For this review, take the finished solid that the model builds, in its own axes (mm). Face numbers are marked on the shaded views. A direction names the side the tool comes from. Coordinates: 2 decimals unless noted, no trailing zeros. Order: outer loops, then holes, each group sorted by start corner. A loop starts at its lowest first (then second) coordinate and runs counter-clockwise, first axis right, second up. Notation, with made-up numbers: (13, 73) -> (50, 73) arc R10 cw to (50, 91) -> close; hole circle Ø3 at (-32, -6). An arc over 180 degrees is marked (long way). Return JSON: item names as keys, results as strings. Group by question number.
Item 1: Machinability: for the marked faces 1, 2, 3, 4 and 5, which of the approach directions +Z, -Z, +X, -X, +Y, -Y give a long, thin tool a straight path to every point of the face, cutting with its end or side? Answer none if there is none.
Item 2: Take a section at B-B (z = 8.5). Write out the cut boundary in (x, y) (3 decimals), then the cut area to 3 significant figures.
Item 3: For line 1 along Y through (x, z) = (-6, 7.1) (3 decimals); line 2 along X through (y, z) = (-5, 7) (3 decimals); line 3 along Z through (x, y) = (-2.5, -3), list the stretches that pass through material, from the lowest coordinate up.
Item 4: Take a section at A-A (x = 0). Write out the cut boundary in (y, z) (3 decimals), then the cut area to 3 significant figures.
Item 5: Insertion check: pin 1 (2 mm diameter, centred on x = -6, z = 6, fed in from -Y) (3 decimals); pin 2 (1.5 mm diameter, centred on x = -3, y = -4.5, fed in from -Z); pin 3 (2 mm diameter, centred on x = 8.5, z = 8, fed in from +Y) (3 decimals); pin 4 (4 mm diameter, centred on x = 8.5, z = 1, fed in from -Y). Each pin has a flat end and moves straight along its axis. Give the tip position at first contact, or say it passes through.
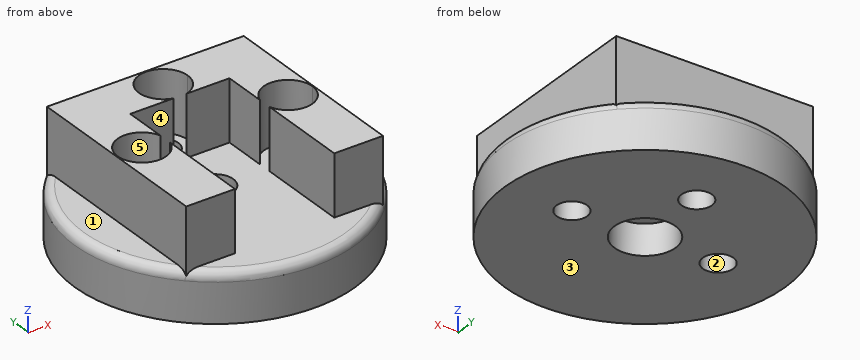
```python
from build123d import *

# Parameters (mm, degrees)
F0_R     = 11.5
F0_R_2   = 1.25
F0_R_3   = 1.5
F1_DEPTH = 4
F3_DEPTH = 5
F5_R     = 2.5
F5_R_2   = 1.5
F6_DEPTH = 2.5


# Not quite as in the source:
# - a fillet or chamfer that OpenCascade refuses, or shapes differently, is made with other operations: its cross-section is extruded or revolved along the edge and cut away or added
# - a feature names something its author has since deleted; it is built from what else it names


with BuildPart() as f1:
    # F0 (on Top) → F1 (new body)
    with BuildSketch(Plane.XY):
        Circle(F0_R)
        with Locations((-6, 0)):
            Circle(F0_R_2, mode=Mode.SUBTRACT)
        Circle(F0_R_3, mode=Mode.SUBTRACT)
        with Locations((6, 0)):
            Circle(F0_R_2, mode=Mode.SUBTRACT)
        with Locations((0, 6)):
            Circle(F0_R_2, mode=Mode.SUBTRACT)
    extrude(amount=F1_DEPTH)

    # F2 (on face) → F3 (join)
    with BuildSketch(Plane.XY.offset(4)):
        with BuildLine():
            Line((0.5425633604, 4.075), (4.075, 4.075))
            Line((4.075, 4.075), (4.075, 0.5425633604))
            ThreePointArc((4.075, 0.5425633604), (6.2738612788, 1.9811612756), (8, 0))
            ThreePointArc((8, 0), (6.2738612788, -1.9811612756), (4.075, -0.5425633604))
            Line((4.075, -0.5425633604), (4.075, -4.075))
            Line((4.075, -4.075), (4.075, -8.075))
            Line((4.075, -8.075), (8.075, -8.075))
            Line((8.075, -8.075), (8.075, 8.075))
            Line((8.075, 8.075), (-8.075, 8.075))
            Line((-8.075, 8.075), (-8.075, -8.075))
            Line((-8.075, -8.075), (-4.075, -8.075))
            Line((-4.075, -8.075), (-4.075, -4.075))
            Line((-4.075, -4.075), (-4.075, -0.5425633604))
            ThreePointArc((-4.075, -0.5425633604), (-8, 0), (-4.075, 0.5425633604))
            Line((-4.075, 0.5425633604), (-4.075, 4.075))
            Line((-4.075, 4.075), (-0.5425633604, 4.075))
            ThreePointArc((-0.5425633604, 4.075), (-1.2072434053, 7.5945417399), (2, 6))
            ThreePointArc((2, 6), (1.5945417399, 4.7927565947), (0.5425633604, 4.075))
        make_face()
    extrude(amount=F3_DEPTH)

    # F4: fillet of radius 0.75 on 1 edges, made by hand


with BuildPart() as f4_tool2:
    # F4_s3 → F4_t4 (revolve)
    with BuildSketch(Plane.XZ):
        with BuildLine():
            ThreePointArc((11.5, 3.25), (11.2803300859, 3.7803300859), (10.75, 4))
            Line((10.75, 4), (11.5, 4))
            Line((11.5, 4), (11.5, 3.25))
        make_face()
    revolve(axis=Axis((0, 0, 4), (0, 0, 1)))

    split(bisect_by=Plane.YZ.offset(8.075), keep=Keep.TOP)


with BuildPart() as f1_1:
    add(f1.part)

    # F4_t1: cut F4_tool2
    add(f4_tool2.part, mode=Mode.SUBTRACT)


with BuildPart() as f4_tool7:
    # F4_s8 → F4_t9 (revolve)
    with BuildSketch(Plane.XZ):
        with BuildLine():
            ThreePointArc((11.5, 3.25), (11.2803300859, 3.7803300859), (10.75, 4))
            Line((10.75, 4), (11.5, 4))
            Line((11.5, 4), (11.5, 3.25))
        make_face()
    revolve(axis=Axis((0, 0, 4), (0, 0, 1)))

    split(bisect_by=Plane.XZ.offset(-8.075), keep=Keep.BOTTOM)


with BuildPart() as f1_2:
    add(f1_1.part)

    # F4_t6: cut F4_tool7
    add(f4_tool7.part, mode=Mode.SUBTRACT)


with BuildPart() as f4_tool12:
    # F4_s13 → F4_t14 (revolve)
    with BuildSketch(Plane.XZ):
        with BuildLine():
            ThreePointArc((11.5, 3.25), (11.2803300859, 3.7803300859), (10.75, 4))
            Line((10.75, 4), (11.5, 4))
            Line((11.5, 4), (11.5, 3.25))
        make_face()
    revolve(axis=Axis((0, 0, 4), (0, 0, 1)))

    split(bisect_by=Plane.XZ.offset(8.075), keep=Keep.TOP)


with BuildPart() as f1_3:
    add(f1_2.part)

    # F4_t11: cut F4_tool12
    add(f4_tool12.part, mode=Mode.SUBTRACT)


with BuildPart() as f4_tool17:
    # F4_s18 → F4_t19 (revolve)
    with BuildSketch(Plane.XZ):
        with BuildLine():
            ThreePointArc((11.5, 3.25), (11.2803300859, 3.7803300859), (10.75, 4))
            Line((10.75, 4), (11.5, 4))
            Line((11.5, 4), (11.5, 3.25))
        make_face()
    revolve(axis=Axis((0, 0, 4), (0, 0, 1)))

    split(bisect_by=Plane.YZ.offset(-8.075), keep=Keep.BOTTOM)


with BuildPart() as f1_4:
    add(f1_3.part)

    # F4_t16: cut F4_tool17
    add(f4_tool17.part, mode=Mode.SUBTRACT)

    # F5 (on face) → F6 (cut)
    with BuildSketch(Plane.XY):
        Circle(F5_R)
        Circle(F5_R_2, mode=Mode.SUBTRACT)
    extrude(amount=F6_DEPTH, mode=Mode.SUBTRACT)


solid = f1_4.part
```
Findings below:
{
 "1": {"face 1": "+Z, -X, +Y, -Y", "face 2": "+Z, -Z", "face 3": "-Z, +X, -X, +Y, -Y", "face 4": "+Z, -Y", "face 5": "+Z"},
 "2": {"outline": "(-8.075, -8.075) -> (-4.075, -8.075) -> (-4.075, -0.543) arc R2 cw (long way) to (-4.075, 0.543) -> (-4.075, 4.075) -> (-0.543, 4.075) arc R2 cw (long way) to (0.543, 4.075) -> (4.075, 4.075) -> (4.075, 0.543) arc R2 cw (long way) to (4.075, -0.543) -> (4.075, -8.075) -> (8.075, -8.075) -> (8.075, 8.075) -> (-8.075, 8.075) -> close", "area": "124 mm2"},
 "3": {"line 1": "y = -8.075 to -2, 2 to 8.075", "line 2": "x = -8.075 to -4.075, 4.075 to 8.075", "line 3": "z = 0 to 4"},
 "4": {"outline": "(-11.5, 0) -> (-2.5, 0) -> (-2.5, 2.5) -> (-1.5, 2.5) -> (-1.5, 4) -> (-10.75, 4) arc R0.75 ccw to (-11.5, 3.25) -> close; (1.5, 2.5) -> (2.5, 2.5) -> (2.5, 0) -> (4.75, 0) -> (4.75, 4) -> (1.5, 4) -> close; (7.25, 0) -> (11.5, 0) -> (11.5, 3.25) arc R0.75 ccw to (10.75, 4) -> (8.075, 4) -> (8.075, 9) -> (8, 9) -> (8, 4) -> (7.25, 4) -> close", "area": "65.1 mm2"},
 "5": {"pin 1": "stops at y = -8.075", "pin 2": "stops at z = 0", "pin 3": "stops at y = 8.075", "pin 4": "stops at y = -9.49"}
}
